Read the model definition and answer for the solid it produces. Units are mm, in the model's axes. Face numbers are marked on the shaded views. A direction names the side the tool comes from. Coordinates: 2 decimals unless noted, no trailing zeros. Loops run counter-clockwise (first coordinate to the right, second up) from the corner with the lowest first, then second, coordinate; pieces in that order, holes last. Notation, with made-up numbers: M 17,67.5 L 68,67.5 A17 ccw 68,85.5 Z; hole C 67.5,-1 d11. An arc over 180 degrees is marked long. One line per item, written item: value. Start each with the question number.
1. For the marked faces 1 and 2, determine the directions among +Z, -Z, +X, -X, +Y, -Y from which every point of the face is accessible in a straight line to the end or side of a thin tool.
2. Determine the mould class of the marked faces 3, 4 and 5 for opening direction X: +X half, -X half, draft (parallel to the pull), parting line (faces both ways), or undercut.
3. The part is cut by section D-D (x = 2.5). Write down the section's boundary in (y, z).
4. Flat-ended cylindrical pins translate along their axes: pin 1 (1 mm diameter, centred on y = 3, z = -7, fed in from -X); pin 2 (1.5 mm diameter, centred on y = 7.5, z = 4.5, fed in from -X). Find the tip coordinate at first contact, or state that the pin passes through.
5. The part is cut by section A-A (x = 7.5). Write down the section's boundary in (y, z).
6. Consider probe 1 along Z at (x, y) = (7.5, 3.75); probe 2 along Y at (x, z) = (2, -4); probe 3 along X at (y, z) = (4.75, 5). Determine where each line is inside the solid, lowest interval first.
7. The part is cut by section C-C (y = 12). Write down the section's boundary in (x, z), then the cut area to 3 significant figures.
8. The part is cut by section B-B (z = 5). Write down the section's boundary in (x, y).
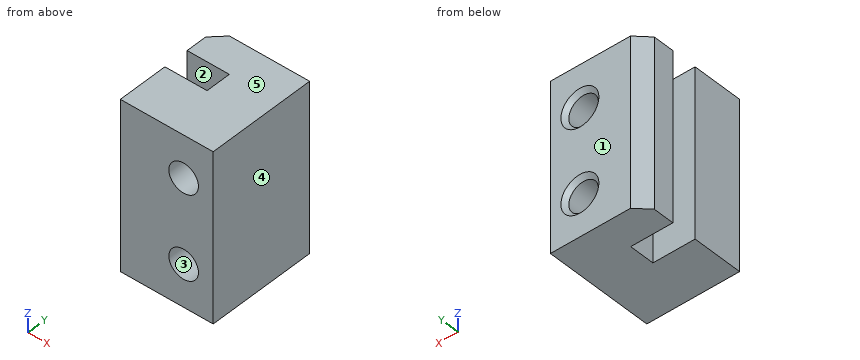
```python
from build123d import *

# Parameters (mm, degrees)
BOSS_EXTRUDE1_DEPTH = 10
SKETCH2_R           = 1.75
CUT_EXTRUDE1_DEPTH  = 14
CHAMFER1_SIZE       = 1.5
SKETCH3_W           = 5
SKETCH3_H           = 13
CUT_EXTRUDE2_DEPTH  = 21
SKETCH4_W           = 20
SKETCH4_H           = 13
BOSS_EXTRUDE2_DEPTH = 1
CHAMFER3_SIZE       = 0.5


with BuildPart() as part:
    # Sketch1 → Boss-Extrude1 (new body, symmetric)
    with BuildSketch(Plane.XY):
        Polygon((0, 0), (15, 0), (15, 6), (10, 6), (10, 9), (15, 9), (15, 13), (0, 13), (0, 9), (5, 9), (5, 6), (0, 6), align=None)
    extrude(amount=BOSS_EXTRUDE1_DEPTH, both=True)

    # Sketch2 → Cut-Extrude1 (cut, through all)
    with BuildSketch(Plane(origin=(0, 13, 0), x_dir=(1, 0, 0), z_dir=(0, 1, 0))):
        with Locations((7.5, -5)):
            Circle(SKETCH2_R)
        with Locations((7.5, 5)):
            Circle(SKETCH2_R)
    extrude(amount=-CUT_EXTRUDE1_DEPTH, mode=Mode.SUBTRACT)

    # Chamfer1
    chamfer1_edges = [part.edges().sort_by_distance(p)[0] for p in [
        (0, 13, 0),
        (15, 13, 0),
    ]]
    chamfer(chamfer1_edges, length=CHAMFER1_SIZE)

    # Sketch3 → Cut-Extrude2 (cut, through all)
    with BuildSketch(Plane.XY.offset(10)):
        with Locations((12.5, 6.5)):
            Rectangle(SKETCH3_W, SKETCH3_H)
    extrude(amount=-CUT_EXTRUDE2_DEPTH, mode=Mode.SUBTRACT)

    # Sketch4 → Boss-Extrude2 (add)
    with BuildSketch(Plane(origin=(10, 0, 0), x_dir=(0, 0, -1), z_dir=(1, 0, 0))):
        with Locations((0, 6.5)):
            Rectangle(SKETCH4_W, SKETCH4_H)
    extrude(amount=BOSS_EXTRUDE2_DEPTH)

    # Chamfer3
    chamfer3_edges = [part.edges().sort_by_distance(p)[0] for p in [
        (5.75, 13, 5),
        (5.75, 13, -5),
    ]]
    chamfer(chamfer3_edges, length=CHAMFER3_SIZE)


solid = part.part
```
Answer block:
1. face 1: +Z, -Z, +X, -X, +Y
1. face 2: +Z, -Z, -X
2. face 3: undercut
2. face 4: +X half
2. face 5: draft
3. outline: M 0,-10 L 6,-10 L 6,10 L 0,10 Z; M 9,-10 L 13,-10 L 13,10 L 9,10 Z
4. pin 1: stops at x = 0
4. pin 2: stops at x = 5
5. outline: M 0,-10 L 13,-10 L 13,-7.25 L 12.5,-6.75 L 0,-6.75 Z; M 0,-3.25 L 12.5,-3.25 L 13,-2.75 L 13,2.75 L 12.5,3.25 L 0,3.25 Z; M 0,6.75 L 12.5,6.75 L 13,7.25 L 13,10 L 0,10 Z
6. probe 1: z = -10 to -6.75, -3.25 to 3.25, 6.75 to 10
6. probe 2: y = 0 to 6, 9 to 13
6. probe 3: x = 0 to 5.75, 9.25 to 11
7. outline: M 0.5,-10 L 11,-10 L 11,10 L 0.5,10 Z; hole C 7.5,-5 d3.5; hole C 7.5,5 d3.5
7. area: 191 mm2
8. outline: M 0,0 L 5.75,0 L 5.75,12.5 L 5.25,13 L 1.5,13 L 0,11.5 L 0,9 L 5,9 L 5,6 L 0,6 Z; M 9.25,0 L 11,0 L 11,13 L 9.75,13 L 9.25,12.5 Z
